from build123d import *

# Parameters (mm, degrees)
SKETCH2_R           = 1.5
BOSS_EXTRUDE3_DEPTH = 6.35


with BuildPart() as part:
    # Sketch2 → Boss-Extrude3 (new body)
    with BuildSketch(Plane.XY):
        Polygon((-5.178463077, 27.016673705), (-5.178463077, 43.486673705), (-5.178463077, 136.886673705), (-5.178463077, 153.356673705), (65.137170919, 153.356673705), (65.137170919, 27.016673705), align=None)
        with Locations((39.821536923, 38.486673705)):
            Circle(SKETCH2_R, mode=Mode.SUBTRACT)
        with Locations((9.821536923, 38.486673705)):
            Circle(SKETCH2_R, mode=Mode.SUBTRACT)
        with Locations((-0.178463077, 38.486673705)):
            Circle(SKETCH2_R, mode=Mode.SUBTRACT)
        with Locations((48.671536923, 38.486673705)):
            Circle(SKETCH2_R, mode=Mode.SUBTRACT)
        with Locations(Location((48.671536923, 141.886673705, 0), (0, 0, 180))):
            Circle(SKETCH2_R, mode=Mode.SUBTRACT)
        with Locations(Location((-0.178463077, 141.886673705, 0), (0, 0, 180))):
            Circle(SKETCH2_R, mode=Mode.SUBTRACT)
        with Locations(Location((9.821536923, 141.886673705, 0), (0, 0, 180))):
            Circle(SKETCH2_R, mode=Mode.SUBTRACT)
        with Locations(Location((39.821536923, 141.886673705, 0), (0, 0, 180))):
            Circle(SKETCH2_R, mode=Mode.SUBTRACT)
    extrude(amount=BOSS_EXTRUDE3_DEPTH)


solid = part.part
Input: part model. Units: mm. Frame: model coordinates. Coordinates: 2 decimals unless noted, no trailing zeros. Loops run counter-clockwise (first coordinate to the right, second up) from the corner with the lowest first, then second, coordinate; pieces in that order, holes last. Notation, with made-up numbers: (15.5, -36) - (33.5, -36) arc R9 cw to (33.5, -31) - close; hole circle Ø3 at (-17, -30). An arc over 180 degrees is marked (long way). Answer in a Markdown table with one row per item. Add a question column.
Item 1: Mould query, pull axis Y, two halves, no side actions, for faces 1 (the flat face through (30, 27.017, 3)), 2 (the cylindrical face through (8.436, 142.461, 3.131)), 3 (the flat face through (65.137, 91, 3)). Classes: released by +Y, released by -Y, zero draft, split by the parting line, or undercut.
Item 2: Contact query for a flat-ended pin moving along its axis: P1, Ø1.8, axis at x = 9.82, y = 38.49, coming from the -Z side. Output: stop coordinate, or through.
Item 3: Line query: line 1 along Y through (x, z) = (-0.5, 5); line 2 along Y through (x, z) = (50, 3). Output: solid intervals per line, ascending. Write a range as [from, to].
Item 4: Section query A-A on x = 48.5. Return the cut outline in (y, z), then the cut area to 3 significant figures.
Recorded:
| question | item | result |
|---|---|---|
| 1 | face 1 | released by -Y |
| 1 | face 2 | undercut |
| 1 | face 3 | zero draft |
| 2 | P1 | through |
| 3 | line 1 | [27.02, 37.02], [39.95, 140.42], [143.35, 153.36] |
| 3 | line 2 | [27.02, 37.79], [39.18, 141.19], [142.58, 153.36] |
| 4 | outline | (27.02, 0) - (37, 0) - (37, 6.35) - (27.02, 6.35) - close; (39.98, 0) - (140.4, 0) - (140.4, 6.35) - (39.98, 6.35) - close; (143.38, 0) - (153.36, 0) - (153.36, 6.35) - (143.38, 6.35) - close |
| 4 | area | 764 mm^2 |
